Here's how the part is built. I have some questions about the finished solid (model axes, mm). Face numbers are marked on the shaded views. Round coordinates to 2 decimals unless told otherwise and drop trailing zeros. Loops run counter-clockwise (first coordinate to the right, second up) from the corner with the lowest first, then second, coordinate; pieces in that order, holes last. Notation, with made-up numbers: (87.25, 13) - (124.25, 13) arc R36 ccw to (124.25, 52) - close; hole circle Ø6 at (68, 2). An arc over 180 degrees is marked (long way). Return JSON: item names as keys, results as strings. Group by question number.
Autodesk Inventor part; units mm, degrees
ref_plane "YZ Plane" through (0, 0, 0) normal (1, 0, 0) x (0, 1, 0)
ref_plane "XZ Plane" through (0, 0, 0) normal (0, 1, 0) x (-1, 0, 0)
ref_plane "XY Plane" through (0, 0, 0) normal (0, 0, 1) x (1, 0, 0)
sketch "Sketch1" plane through (0, 0, 0) normal (0, 1, 0) x (-1, 0, 0)
  line L0 (43.4289, -18.5999) -> (-45.4711, -18.5999)
  line L1 (-45.4711, -18.5999) -> (-45.4711, 24.5801)
  line L2 (-45.4711, 24.5801) -> (43.4289, 24.5801)
  line L3 (43.4289, 24.5801) -> (43.4289, -18.5999)
  point P0 (0, 0)
  dimension "d2" = 88.9
  dimension "d3" = 43.18
extrude "Extrusion1" add sketch "Sketch1" along normal blind 6.35
sketch "Sketch2" plane through (0, 6.35, 0) normal (0, 1, 0) x (1, 0, 0)
  point P0 (0, 0)
  point P1 (-0.0268, -24.5835)
hole "Hole1" at (-0.0268, 6.35, 24.5835) direction (0, -1, 0) diameter 41.148 end through all
properties part number "InventorPart1Commit2"
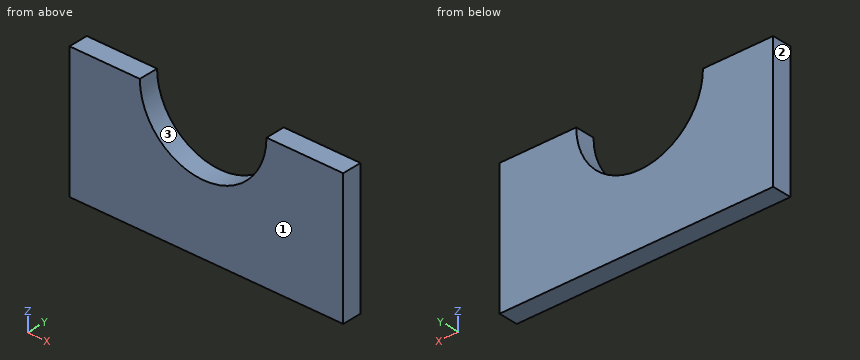
Q1. If we mould it in two halves opening along X, with no side actions, what happens to the marked faces 1, 2 and 3? For each: +X half, -X half, draft (parallel to the pull), parting line (faces both ways), or undercut.
Q2. Imagine slicing it at B-B, the plane y = 3. List the corners of the cut face in (x, z) for me, and give its area (3 significant figures).
Q3. Imagine slicing it at D-D, the plane x = -9.5. List the corners of the cut face in (y, z) for me.
Q4. Please list where these lines run through material, in increasing order: line 1 (Z direction, x = 0, y = 5); line 2 (X direction, y = 1.25, z = 17); line 3 (X direction, y = 1.25, z = 6).
Q5. Imagine slicing it at C-C, the plane x = 16. List the corners of the cut face in (y, z) for me.
Q6. Imagine slicing it at A-A, the plane z = 19.5. List the corners of the cut face in (x, y) for me.
Output values:
{
 "1": {"face 1": "draft", "face 2": "-X half", "face 3": "undercut"},
 "2": {"outline": "(-43.43, -18.6) - (45.47, -18.6) - (45.47, 24.58) - (20.55, 24.58) arc R20.57 cw to (-20.6, 24.58) - (-43.43, 24.58) - close", "area": "3,170 mm^2"},
 "3": {"outline": "(0, -18.6) - (6.35, -18.6) - (6.35, 6.32) - (0, 6.32) - close"},
 "4": {"line 1": "z = -18.6 to 4.01", "line 2": "x = -43.43 to -19.15, 19.1 to 45.47", "line 3": "x = -43.43 to -8.86, 8.8 to 45.47"},
 "5": {"outline": "(0, -18.6) - (6.35, -18.6) - (6.35, 11.68) - (0, 11.68) - close"},
 "6": {"outline": "(-43.43, 0) - (-19.96, 0) - (-19.96, 6.35) - (-43.43, 6.35) - close; (19.91, 0) - (45.47, 0) - (45.47, 6.35) - (19.91, 6.35) - close"}
}
